Design review of the part shown in the three views and the two pictorial views. Dimensions are in mm from the part's minimum x, y and z. Coordinates: 2 decimals unless noted, no trailing zeros. Loops run counter-clockwise (first coordinate to the right, second up) from the corner with the lowest first, then second, coordinate; pieces in that order, holes last.
Q1. For P1, Ø1.8, axis at x = 2.66, y = 2.66, coming from the -Z side, flat-tipped, find the tip position at first contact; note if it passes through.
Q2. Add section C-C on x = 20.75. Give the boundary of the cut face in (y, z), and give its area (3 significant figures).
Q3. Add section A-A on y = 11.5. Give the boundary of the cut face in (x, z).
Q4. Add section D-D on z = 0.4. Give the boundary of the cut face in (x, y).
Q5. Wall thickness on probe 1 along Y at (x, z) = (11.5, 0.2); probe 2 along X at (y, z) = (19.25, 0.5); probe 3 along X at (y, z) = (19, 0.95) (1 decimal): over which ranges is each line inside the solid? List them lowest first.
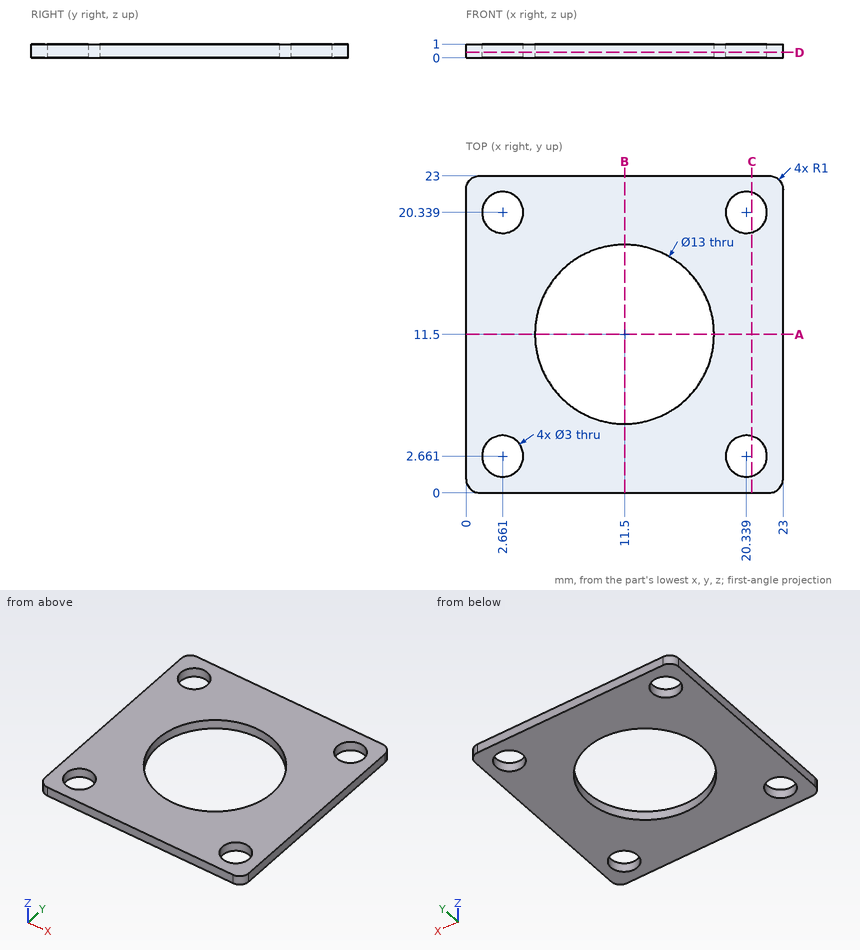
Entries:
1. P1: passes through
2. outline: (0, 0) - (1.22, 0) - (1.22, 1) - (0, 1) - close; (4.1, 0) - (18.9, 0) - (18.9, 1) - (4.1, 1) - close; (21.78, 0) - (23, 0) - (23, 1) - (21.78, 1) - close
2. area: 17.2 mm2
3. outline: (0, 0) - (5, 0) - (5, 1) - (0, 1) - close; (18, 0) - (23, 0) - (23, 1) - (18, 1) - close
4. outline: (0, 1) arc R1 ccw to (1, 0) - (22, 0) arc R1 ccw to (23, 1) - (23, 22) arc R1 ccw to (22, 23) - (1, 23) arc R1 ccw to (0, 22) - close; hole circle Ø3 at (2.66, 2.66); hole circle Ø3 at (2.66, 20.34); hole circle Ø13 at (11.5, 11.5); hole circle Ø3 at (20.34, 2.66); hole circle Ø3 at (20.34, 20.34)
5. probe 1: y = 0 to 5, 18 to 23
5. probe 2: x = 0 to 1.63, 3.69 to 19.31, 21.37 to 23
5. probe 3: x = 0 to 2, 3.3 to 19.7, 21 to 23
